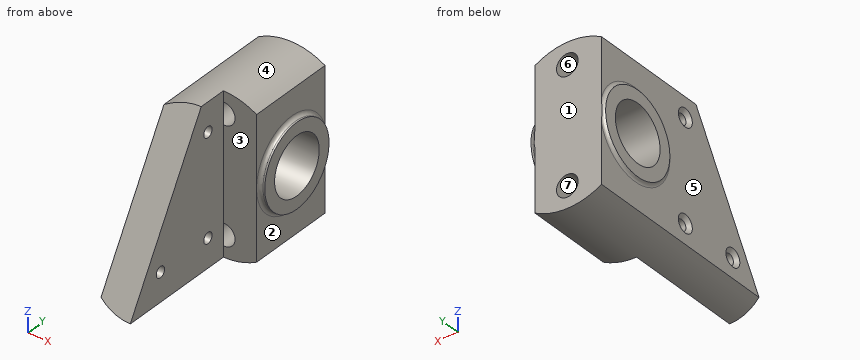
Autodesk Inventor part; units mm, degrees
ref_plane "Arbeitsebene1" through (0, 45.8, 0) normal (0, 1, 0) x (-1, 0, 0)
ref_plane "Arbeitsebene2" through (0, 45.8, 0) normal (0, 1, 0) x (-1, 0, 0)
ref_plane "Arbeitsebene3" through (0, 0, 0) normal (1, 0, 0) x (0, 1, 0)
sketch "Skizze1" plane through (0, 0, 0) normal (0, 1, 0) x (-1, 0, 0)
  line L0 (9.25, 16.0215) -> (9.25, -23.0215)
  line L1 (-9.25, 16.0215) -> (-9.25, -23.0215)
  arc A0 (-9.25, -23.0215) -> (9.25, -23.0215) centre (0, -7) ccw
  arc A1 (9.25, 16.0215) -> (-9.25, 16.0215) centre (0, 0) ccw
  line L2 (9.25, -3.5) -> (-9.25, -3.5) construction
  line L3 (0, 18.5) -> (0, -26.5698) construction
  point P0 (0, -25.5)
  dimension "d1" = 18.5
  dimension "d2" = 44
  dimension "d3" = 18.5
extrude "Extrusion1" add sketch "Skizze1" along normal blind 57.8
sketch "Skizze2" plane through (9.25, 0, 16.0215) normal (1, 0, 0) x (0, 0, -1)
  line L0 (0, 0) -> (-2.4785, 0)
  line L1 (41.5215, 0) -> (41.5215, 57.8)
  line L2 (0, 0) -> (39.0429, 0)
  line L3 (41.5215, 0) -> (39.0429, 0)
  line L4 (-2.4785, 0) -> (-2.4785, 57.8)
  line L5 (41.5215, 0) -> (-2.4785, 25.4034)
  point P0 (16.0215, 0)
  dimension "d143" = 60
extrude "Extrusion2" cut sketch "Skizze2" against normal up to surface (18.5 mm away)
ref_plane "Arbeitsebene1" through (0, 45.8, 0) normal (0, 1, 0) x (-1, 0, 0)
sketch "Skizze8" plane through (-9.25, 57.8, -23.0215) normal (-1, 0, 0) x (0, 0, 1)
  circle A0 centre (19.5215, -12) radius 11.5
  line L0 (0, 0) -> (39.0429, 0)
  point P0 (23.0215, -57.8)
  point P1 (19.5215, 0)
  dimension "d40" = 23
  dimension "d41" = 12
extrude "Extrusion5" add sketch "Skizze8" along normal mid plane 1.5
sketch "Skizze9" plane through (9.25, 57.8, 16.0215) normal (1, 0, 0) x (0, 0, -1)
  circle A0 centre (19.5215, -12) radius 11.5
  line L0 (0, 0) -> (39.0429, 0)
  point P0 (16.0215, -57.8)
  point P1 (19.5215, 0)
  dimension "d44" = 23
  dimension "d45" = 12
extrude "Extrusion6" add sketch "Skizze9" along normal blind 1.5
sketch "Skizze10" plane through (10.75, 45.8, -3.5) normal (1, 0, 0) x (0, 0, -1)
  circle A0 centre (0, 0) radius 11.5
  point P0 (-3.5, -45.8)
hole "Bohrung4" at (10.75, 45.8, -3.5) direction (-1, 0, 0) diameter 16 depth 20.75
ref_plane "Arbeitsebene2" through (0, 45.8, 0) normal (0, 1, 0) x (-1, 0, 0)
split_face "Trennen2"
sketch "Skizze11" plane through (0, 57.8, 0) normal (0, 1, 0) x (1, 0, 0)
  line L0 (0, 0) -> (5.4139, 0) construction
  arc A0 (-9.25, -16.0215) -> (9.25, -16.0215) centre (0, 0) ccw
  line L1 (0, -18.5) -> (0, 25.5) construction
  arc A1 (9.25, 23.0215) -> (-9.25, 23.0215) centre (0, 7) ccw
  point P0 (0, -12.5)
  point P1 (0, 19.5)
  point P2 (0, 3.5)
  dimension "d67" = 16
  dimension "d68" = 32
ref_plane "Arbeitsebene3" through (0, 0, 0) normal (1, 0, 0) x (0, 1, 0)
fillet "Rundung1" radius 1 2 edges at (9.25, 45.8, 8) (-9.25, 45.8, -15)
sketch "Skizze17" plane through (0, 0, 0) normal (1, 0, 0) x (0, 1, 0)
  line L0 (0, -25.5) -> (45.8, -25.5)
  arc A0 (45.8, -11.5) -> (45.8, 4.5) centre (45.8, -3.5) ccw
  arc A1 (45.8, 4.5) -> (45.8, -11.5) centre (45.8, -3.5) ccw
  arc A2 (45.8, 4.5) -> (45.8, -11.5) centre (45.8, -3.5) ccw
  line L1 (57.8, -0.1152) -> (57.8, 16.0215)
  point P0 (0, 0)
  point P1 (68.19, 2.5)
  dimension "d112" = 10.39
  dimension "d113" = 6
ref_plane "Arbeitsebene8" through (0, 0, 19) normal (0, 0, 1) x (1, 0, 0)
sketch "Skizze22" plane through (0, 0, 19) normal (0, 0, 1) x (1, 0, 0)
  line L0 (-9.25, 45.8) -> (-9.25, 33.3318)
  line L1 (0, 0) -> (9.5, 0)
  line L2 (9.5, 0) -> (9.5, 33.3318)
  line L3 (9.5, 33.3318) -> (0, 33.3318)
  line L4 (0, 33.3318) -> (0, 0)
  dimension "d125" = 9.5
extrude "Extrusion8" cut sketch "Skizze22" against normal through all
sketch "Skizze25" plane through (-9.25, 1.431, -23.0215) normal (-1, 0, 0) x (0, 0, 1)
  line L0 (-2.4785, 31.9008) -> (-2.4785, -1.431)
  arc A0 (11.5215, 44.369) -> (27.5215, 44.369) centre (19.5215, 44.369) ccw
  arc A1 (27.5215, 44.369) -> (11.5215, 44.369) centre (19.5215, 44.369) ccw
  point P0 (23.0215, -1.431)
  point P1 (5.5215, 9.369)
  point P2 (5.5215, 26.369)
  point P3 (33.5215, 26.369)
  dimension "d144" = 10.8
  dimension "d145" = 14
  dimension "d146" = 17
  dimension "d147" = 14
hole "Bohrung11" at (-9.25, 10.8, -17.5) at (-9.25, 27.8, -17.5) at (-9.25, 27.8, 10.5) direction (1, 0, 0) diameter 3 depth 9.25 countersink diameter 5 countersink angle 90
sketch "Skizze26" plane through (0, 57.8, 0) normal (0, 1, 0) x (1, 0, 0)
  line L0 (0, 25.5) -> (0, -18.5)
  line L1 (-9.25, 23.0215) -> (-9.25, 6.8848)
  line L2 (-9.25, 0.1152) -> (-9.25, -16.0215)
  line L3 (9.25, 7) -> (9.25, 23.0215)
  line L4 (9.25, -16.0215) -> (9.25, 0)
  arc A0 (9.25, 23.0215) -> (-9.25, 23.0215) centre (0, 7) ccw
  arc A1 (-9.25, -16.0215) -> (9.25, -16.0215) centre (0, 0) ccw
  point P0 (0.25, 19.5)
  point P1 (0.25, -12.5)
  point P2 (0, 25.5)
  point P3 (0, -18.5)
  dimension "d155" = 9.5
  dimension "d156" = 9.5
  dimension "d157" = 6
  dimension "d158" = 6
hole "Bohrung12" at (0.25, 57.8, 12.5) at (0.25, 57.8, -19.5) direction (0, -1, 0) diameter 6 depth 24.4682
properties part number "1042"
Model file for the job. Use its own axes, mm. Face numbers are marked on the shaded views. A direction names the side the tool comes from. Give positions to 0.01 mm unless a question says otherwise; leave off trailing zeros. Loops run counter-clockwise (first coordinate to the right, second up) from the corner with the lowest first, then second, coordinate; pieces in that order, holes last.
1) Saw through at B-B (y = 27.8). Write the cut outline in (x, z), plus the area to 3 significant figures.
2) Pull direction X, two halves, no side cores. Call the marked faces 4, 5, 6 and 7: +X half, -X half, draft (parallel to the pull), parting line (faces both ways), or undercut.
3) Saw through at C-C (z = -3.5). Write the cut outline in (x, y), plus the area to 3 significant figures.
4) Saw through at D-D (x = -2). Write the cut outline in (y, z).
5) Saw through at A-A (y = 45.8). Write the cut outline in (x, z), plus the area to 3 significant figures.
6) Tool access for the marked faces 1, 2 and 3: list every direction of +Z, -Z, +X, -X, +Y, -Y with a clear straight run to the whole face (end or side of a thin tool).
7) Flat gauge pins, fed straight in: pin 1 Ø1 at (x, z) = (-5, 2) entering from -Y; pin 2 Ø2 at (x, z) = (-1.5, 12.5) entering from +Y; pin 3 Ø2.5 at (y, z) = (10.8, -17.5) entering from +X; pin 4 Ø2 at (x, y) = (-7.5, 7) entering from +Z. Where does each tip first touch, or does it go through?
8) Wall check: line 1 (X direction, y = 51.5, z = -19.5); line 2 (Z direction, x = 0.25, y = 46.5); line 3 (Y direction, x = -8.5, z = -18). Give the ranges that are in metal, low to high.
Answer block:
1. outline: (-9.25, -23.02) arc R18.5 ccw to (0, -25.5) - (0, -19) - (-8.25, -19) - (-9.25, -20) - close; (-9.25, -15) - (-8.25, -16) - (0, -16) - (0, 9) - (-8.25, 9) - (-9.25, 8) - close; (-9.25, 13) - (-8.25, 12) - (0, 12) - (0, 18.5) arc R18.5 ccw to (-9.25, 16.02) - close
1. area: 335 mm2
2. face 4: parting line
2. face 5: -X half
2. face 6: undercut
2. face 7: undercut
3. outline: (-10, 34.3) arc R1 cw to (-9.25, 33.33) - (-9.25, 12.7) - (0, 12.7) - (0, 33.33) - (9.25, 33.33) arc R1 cw to (10.25, 34.3) - (10.75, 34.3) - (10.75, 37.8) - (-10, 37.8) - close; (-10, 53.8) - (10.75, 53.8) - (10.75, 57.3) - (10.25, 57.3) arc R1 cw to (9.38, 57.8) - (-9.37, 57.8) arc R1 cw to (-10, 57.3) - close
3. area: 364 mm2
4. outline: (0.06, -25.39) - (57.8, -25.39) - (57.8, -21.48) - (33.33, -21.48) - (33.33, -17.52) - (57.8, -17.52) - (57.8, 10.52) - (33.33, 10.52) - (33.33, 14.48) - (57.8, 14.48) - (57.8, 18.39) - (25.34, 18.39) - close; hole circle Ø3 at (10.8, -17.5); hole circle Ø3 at (27.8, -17.5); hole circle Ø3 at (27.8, 10.5); hole circle Ø16 at (45.8, -3.5)
5. outline: (-10, -15) arc R1 cw to (-9.25, -15.97) - (-9.25, -23.02) arc R18.5 ccw to (9.25, -23.02) - (9.25, -16) arc R1 cw to (10.25, -15) - (10.75, -15) - (10.75, -11.5) - (-10, -11.5) - close; (-10, 4.5) - (10.75, 4.5) - (10.75, 8) - (10.25, 8) arc R1 cw to (9.25, 9) - (9.25, 16.02) arc R18.5 ccw to (-9.25, 16.02) - (-9.25, 8.97) arc R1 cw to (-10, 8) - close; hole circle Ø6 at (0.25, -19.5); hole circle Ø6 at (0.25, 12.5)
5. area: 448 mm2
6. face 1: +Z, -Z, +X, -X, +Y
6. face 2: -Z, +X
6. face 3: +Z, -Z, +X, -Y
7. pin 1: stops at y = 15.59
7. pin 2: stops at y = 33.33
7. pin 3: passes through
7. pin 4: stops at z = -11.64
8. line 1: x = -9.25 to -2.75, 3.25 to 9.25
8. line 2: z = -25.5 to -22.5, -16.5 to -11.47, 4.47 to 9.5, 15.5 to 18.5
8. line 3: y = 4.33 to 9.12, 12.48 to 26.12, 29.48 to 57.8
